Autodesk Inventor part; units mm, degrees
ref_plane "YZ Plane" through (0, 0, 0) normal (1, 0, 0) x (0, 1, 0)
ref_plane "XZ Plane" through (0, 0, 0) normal (0, 1, 0) x (-1, 0, 0)
ref_plane "XY Plane" through (0, 0, 0) normal (0, 0, 1) x (1, 0, 0)
sketch "スケッチ1" plane through (0, 0, 0) normal (0, 0, 1) x (1, 0, 0)
  circle A0 centre (0, 0) radius 10.5 construction
  line L0 (0, 10.5) -> (-162.5, 10.5) construction
  line L1 (-162.5, 10.5) -> (-162.5, -10.5) construction
  line L2 (-162.5, -10.5) -> (0, -10.5) construction
  circle A1 centre (-157.5, 0) radius 1.55 construction
  line L3 (-147.5, 2.5) -> (-32.5, 2.5) construction
  line L4 (-32.5, 2.5) -> (-32.5, -2.5) construction
  line L5 (-32.5, -2.5) -> (-147.5, -2.5) construction
  line L6 (-147.5, -2.5) -> (-147.5, 2.5) construction
  line L7 (-90, 2.5) -> (-90, -2.5) construction
  circle A2 centre (-22.5, 0) radius 1.55 construction
  line L8 (-12, 21.3027) -> (-12, -27.3903) construction
  line L9 (-32.45, 2.55) -> (-147.55, 2.55) construction
  line L10 (-147.55, 2.55) -> (-147.55, -2.55) construction
  line L11 (-147.55, -2.55) -> (-32.45, -2.55) construction
  line L12 (-32.45, -2.55) -> (-32.45, 2.55) construction
  circle A3 centre (-146.5, 2.55) radius 1.05 construction
  line L13 (-147.5, 0) -> (-90, 0) construction
  line L14 (-147.55, 2.55) -> (-147.55, -2.55) construction
  arc A4 (-145.45, 2.55) -> (-147.55, 2.55) centre (-146.5, 2.55) ccw construction
  line L15 (-145.45, 2.55) -> (-34.55, 2.55) construction
  arc A5 (-32.45, 2.55) -> (-34.55, 2.55) centre (-33.5, 2.55) ccw construction
  line L16 (-32.45, 2.55) -> (-32.45, -2.55) construction
  arc A6 (-147.55, -2.55) -> (-145.45, -2.55) centre (-146.5, -2.55) ccw construction
  line L17 (-145.45, -2.55) -> (-34.55, -2.55) construction
  arc A7 (-34.55, -2.55) -> (-32.45, -2.55) centre (-33.5, -2.55) ccw construction
  circle A8 centre (0, 8.5) radius 1.35
  circle A9 centre (0, 0) radius 5.05
  circle A10 centre (-8.5, 0) radius 1.35
  circle A11 centre (0, -8.5) radius 1.35
  circle A12 centre (8.5, 0) radius 1.35
  line L18 (-162.5, 4.8006) -> (-162.5, -4.8006) construction
  line L19 (-162.5, 4.8006) -> (-22.5, 10.5) construction
  line L20 (-22.5, 10.5) -> (0, 10.5) construction
  line L21 (-162.5, -4.8006) -> (-22.5, -10.5) construction
  line L22 (-22.5, -10.5) -> (0, -10.5) construction
  arc A13 (0, -10.5) -> (0, 10.5) centre (0, 0) ccw construction
  circle A14 centre (-157.5, 0) radius 5 construction
  circle A15 centre (-21.5, 0) radius 1.55
  circle A16 centre (-46.5, 0) radius 1.55
  line L23 (-17.5, -2.5) -> (-50.5, -2.5) construction
  line L24 (-50.5, -2.5) -> (-50.5, 2.5) construction
  line L25 (-50.5, 2.5) -> (-17.5, 2.5) construction
  line L26 (-17.5, 2.5) -> (-17.5, -2.5) construction
  line L27 (-27.5, -2.5) -> (-40.5, -2.5) construction
  line L28 (-40.5, -2.5) -> (-40.5, 2.5) construction
  line L29 (-40.5, 2.5) -> (-27.5, 2.5) construction
  line L30 (-27.5, 2.5) -> (-27.5, -2.5) construction
  line L31 (-27.45, -2.55) -> (-40.55, -2.55)
  line L32 (-40.55, -2.55) -> (-40.55, 2.55)
  line L33 (-40.55, 2.55) -> (-27.45, 2.55)
  line L34 (-27.45, 2.55) -> (-27.45, -2.55)
  circle A17 centre (-28.5, -2.55) radius 1.05
  circle A18 centre (-28.5, 2.55) radius 1.05
  circle A19 centre (-39.5, -2.55) radius 1.05
  circle A20 centre (-39.5, 2.55) radius 1.05
  line L35 (-50.5, 2.5) -> (-50.5, -2.5)
  line L36 (-50.5, -2.5) -> (-16.9113, -10.5)
  line L37 (-50.5, 2.5) -> (-16.9113, 10.5)
  arc A21 (0, -10.5) -> (0, 10.5) centre (0, 0) ccw
  line L38 (-16.9113, 10.5) -> (0, 10.5)
  line L39 (0, -10.5) -> (-16.9113, -10.5)
  circle A22 centre (-39.5, 2.55) radius 2.5 construction
  circle A23 centre (0, 0) radius 16 construction
  circle A24 centre (0, 0) radius 21 construction
  line L40 (-21, 19.3585) -> (-21, -28.09) construction
  point P0 (-162.5, 0)
  point P1 (-17.5, 0)
  dimension "d9" = 2.1
  dimension "d29" = 2.1
  dimension "d0" = 162.5
  dimension "d1" = 3.1
  dimension "d2" = 21
  dimension "d3" = 10
  dimension "d4" = 5
  dimension "d5" = 12
  dimension "d6" = 135
  dimension "d7" = 5
  dimension "d8" = 0.05
  dimension "d10" = 2.7
  dimension "d11" = 8.5
  dimension "d12" = 10.1
  dimension "d15" = 360
  dimension "d20" = 3.1
  dimension "d21" = 5
  dimension "d22" = 4
  dimension "d23" = 5
  dimension "d24" = 25
  dimension "d26" = 10
  dimension "d27" = 4
  dimension "d28" = 10
  dimension "d30" = 0.05
  dimension "d32" = 5
  dimension "d33" = 32
  dimension "d34" = 5
extrude "押し出し1" add sketch "スケッチ1" along normal blind 2
fillet "フィレット2" radius 2 2 edges at (-50.5, 2.5, 1) (-50.5, -2.5, 1)
sketch "スケッチ2" plane through (0, 0, 0) normal (0, 0, -1) x (-1, 0, 0)
  circle A0 centre (0, -8.5) radius 1.35
  circle A1 centre (0, -8.5) radius 1.35
  circle A2 centre (8.5, 0) radius 1.35
  circle A3 centre (8.5, 0) radius 1.35
  circle A4 centre (0, 8.5) radius 1.35
  circle A5 centre (0, 8.5) radius 1.35
  circle A6 centre (-8.5, 0) radius 1.35
  circle A7 centre (-8.5, 0) radius 1.35
  circle A8 centre (21.5, 0) radius 1.55
  circle A9 centre (21.5, 0) radius 1.55
  circle A10 centre (46.5, 0) radius 1.55
  circle A11 centre (46.5, 0) radius 1.55
  point P0 (0, 0)
extrude "押し出し2" add sketch "スケッチ2" against normal up to surface (2 mm away)
equation "\"d2\" = d2_1"
equation "\"d3\" = d3_1"
equation "\"d4\" = d4_1"
equation "\"d6\" = d6_1"
equation "\"d21\" = d4"
equation "\"d27\" = d22"
equation "\"d28\" = d26"
properties part number "前腕_メインフレーム_1_1" material "GFRP"
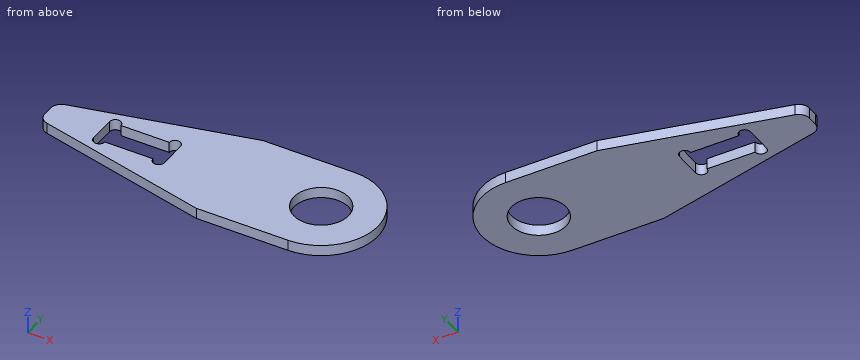
Could you check a few things on this model? Use its own coordinates, in mm. Give positions to 0.01 mm unless a question says otherwise; leave off trailing zeros. Order: outer loops, then holes, each group sorted by start corner. A loop starts at its lowest first (then second) coordinate and runs counter-clockwise, first axis right, second up. Notation, with made-up numbers: (48.5, 51) - (93.5, 51) arc R21 ccw to (93.5, 86) - close; hole circle Ø11 at (-13.5, -25.75). An arc over 180 degrees is marked (long way). Return JSON: item names as keys, results as strings. Group by question number.
Q1. Suppose I cut it at B-B, the plane x = -28.5. Please give me the cut outline in (y, z), and give its area (3 significant figures).
Q2. Will this pin go through, and if not, where does the flat tip stop? pin 1 Ø3 at (x, y) = (-38, 5) entering from -Z.
Q3. Please list where these lines run through material, in increasing order: line 1 along Y through (x, z) = (0, 1.2); line 2 along X through (y, z) = (0.5, 0.55); line 3 along X through (y, z) = (-2.5, 0.4). Write a range as [from, to].
Q4. Suppose I cut it at D-D, the plane x = -1.5. Please give me the cut outline in (y, z).
Q5. Suppose I cut it at C-C, the plane y = 0. Please give me the cut outline in (x, z).
Q6. Suppose I cut it at A-A, the plane z = 0.4. Please give me the cut outline in (x, y).
Resolved:
{
 "1": {"outline": "(-7.74, 0) - (-3.6, 0) - (-3.6, 2) - (-7.74, 2) - close; (3.6, 0) - (7.74, 0) - (7.74, 2) - (3.6, 2) - close", "area": "16.6 mm2"},
 "2": {"pin 1": "stops at z = 0"},
 "3": {"line 1": "y = [-10.5, -5.05], [5.05, 10.5]", "line 2": "x = [-50.5, -40.55], [-27.45, -5.03], [5.03, 10.49]", "line 3": "x = [-49.73, -40.55], [-27.45, -4.39], [4.39, 10.2]"},
 "4": {"outline": "(-10.5, 0) - (-4.82, 0) - (-4.82, 2) - (-10.5, 2) - close; (4.82, 0) - (10.5, 0) - (10.5, 2) - (4.82, 2) - close"},
 "5": {"outline": "(-50.5, 0) - (-40.55, 0) - (-40.55, 2) - (-50.5, 2) - close; (-27.45, 0) - (-5.05, 0) - (-5.05, 2) - (-27.45, 2) - close; (5.05, 0) - (10.5, 0) - (10.5, 2) - (5.05, 2) - close"},
 "6": {"outline": "(-50.5, -0.92) arc R2 ccw to (-48.96, -2.87) - (-16.91, -10.5) - (0, -10.5) arc R10.5 ccw to (0, 10.5) - (-16.91, 10.5) - (-48.96, 2.87) arc R2 ccw to (-50.5, 0.92) - close; hole (-40.55, -2.55) arc R1.05 ccw to (-38.45, -2.55) - (-29.55, -2.55) arc R1.05 ccw to (-27.45, -2.55) - (-27.45, 2.55) arc R1.05 ccw to (-29.55, 2.55) - (-38.45, 2.55) arc R1.05 ccw to (-40.55, 2.55) - close; hole circle Ø10.1 at (0, 0)"}
}
